Check sheet for the drawn part. Datum: minimum x, y, z corner. Units: mm. A direction names the side the tool comes from. Round coordinates to 2 decimals unless told otherwise and drop trailing zeros. Write each loop counter-clockwise with the first axis right and the second up, starting at its lowest first coordinate (ties: lowest second). Pieces come first, ordered by that corner, then holes. Notation, with made-up numbers: M 76,87 L 108,87 A33 ccw 108,123 Z; hole C -38,44.5 d6. An arc over 180 degrees is marked long. Use a Markdown table: item, result.
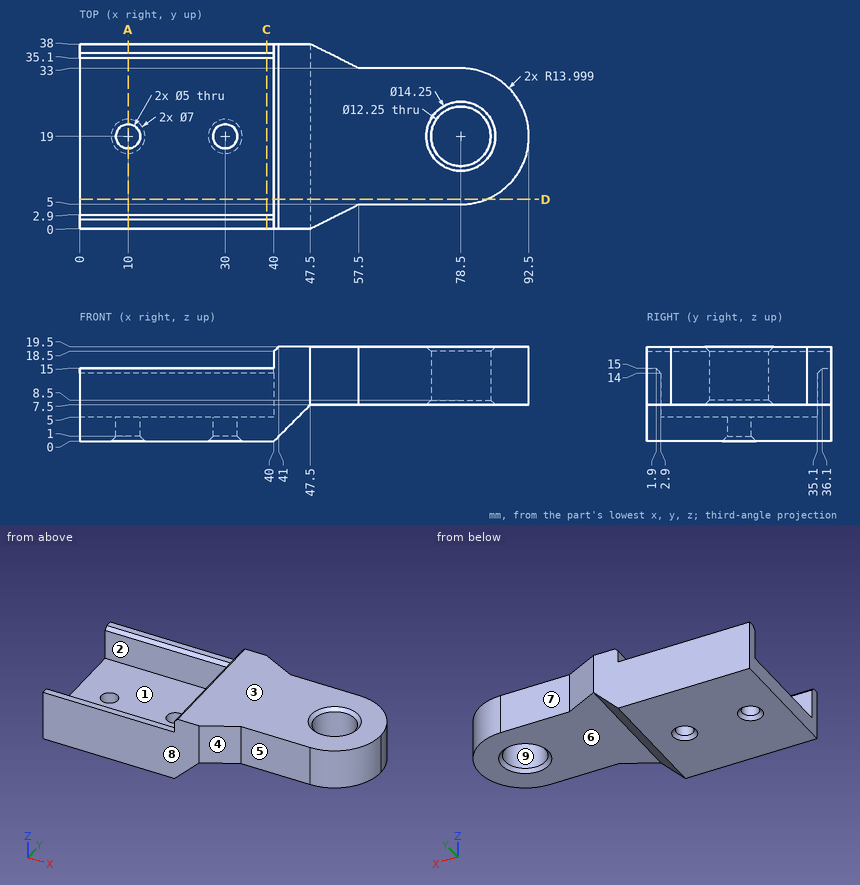
Item 1: Cross-section at C-C, the plane x = 38.5. Record the cut outline in (y, z).
Outcome:
| item | result |
|---|---|
| outline | M 0,0 L 38,0 L 38,15 L 36.1,15 L 35.1,14 L 35.1,5 L 2.9,5 L 2.9,14 L 1.9,15 L 0,15 Z |
Item 2: Material ranges on line 1 along X through (y, z) = (19, 11.25) (1 decimal); line 2 along Y through (x, z) = (30, 3); line 3 along X through (y, z) = (19, 2.25), recorded low to high. Write a range as from..to.
Outcome:
| item | result |
|---|---|
| line 1 | x = 40..72.4, 84.6..92.5 |
| line 2 | y = 0..16.5, 21.5..38 |
| line 3 | x = 0..7.5, 12.5..27.5, 32.5..42.25 |
Item 3: Go/stop test with flat-tipped pins: pin 1 (4 mm diameter, centred on x = 62, z = 8, fed in from -Y); pin 2 (4 mm diameter, centred on y = 14.5, z = 12, fed in from -X); pin 3 (2 mm diameter, centred on y = 25, z = 16, fed in from +X). Record where each tip stops, or that it passes through.
Outcome:
| item | result |
|---|---|
| pin 1 | stops at y = 5 |
| pin 2 | stops at x = 40 |
| pin 3 | stops at x = 91.58 |
Item 4: Cross-section at A-A, the plane x = 10. Record the cut outline in (y, z).
Outcome:
| item | result |
|---|---|
| outline | M 0,0 L 15.5,0 L 16.5,1 L 16.5,5 L 2.9,5 L 2.9,14 L 1.9,15 L 0,15 Z; M 21.5,1 L 22.5,0 L 38,0 L 38,15 L 36.1,15 L 35.1,14 L 35.1,5 L 21.5,5 Z |
Item 5: Cross-section at D-D, the plane y = 6. Record the cut outline in (x, z), and give its area (3 significant figures).
Outcome:
| item | result |
|---|---|
| outline | M 0,0 L 40,0 L 47.5,7.5 L 83.7,7.5 L 83.7,19.5 L 41,19.5 L 40,18.5 L 40,5 L 0,5 Z |
| area | 752 mm2 |
Item 6: Access from +Z, -Z, +X, -X, +Y, -Y to the whole of each face (thin tool, end or side, straight path). Record for the marked faces 5, 6, 7, 8 and 9.
Outcome:
| item | result |
|---|---|
| face 5 | +Z, -Z, +X, -Y |
| face 6 | -Z, +X, +Y, -Y |
| face 7 | +Z, -Z, +X, +Y |
| face 8 | +Z, -Z, +X, -X, -Y |
| face 9 | +Z, -Z |
Item 7: Mould release check, pull along Y, two halves, no side actions. Record for the marked faces 1, 2, 3 and 4: +Y half, -Y half, draft (parallel to the pull), parting line (faces both ways), or undercut.
Outcome:
| item | result |
|---|---|
| face 1 | undercut |
| face 2 | undercut |
| face 3 | draft |
| face 4 | -Y half |
